```python
from build123d import *

# Parameters (mm, degrees)
SKETCH1_R           = 40
BOSS_EXTRUDE1_DEPTH = 10
SKETCH2_R           = 10
BOSS_EXTRUDE2_DEPTH = 500
SKETCH3_R           = 10
BOSS_EXTRUDE3_DEPTH = 30


with BuildPart() as part:
    # Sketch1 → Boss-Extrude1 (new body)
    with BuildSketch(Plane.XY):
        Circle(SKETCH1_R)
    extrude(amount=BOSS_EXTRUDE1_DEPTH)

    # Sketch2 → Boss-Extrude2 (add)
    with BuildSketch(Plane.XY.offset(10)):
        Circle(SKETCH2_R)
    extrude(amount=BOSS_EXTRUDE2_DEPTH)

    # Sketch3 → Boss-Extrude3 (add)
    with BuildSketch(Plane(origin=(0, 0, 0), x_dir=(-1, 0, 0), z_dir=(0, 0, -1))):
        with Locations((26.998561916, 0)):
            Circle(SKETCH3_R)
    extrude(amount=BOSS_EXTRUDE3_DEPTH)


solid = part.part
```
Model file for the job. Use its own axes, mm. A direction names the side the tool comes from. Coordinates: 2 decimals unless noted, no trailing zeros. Order: outer loops, then holes, each group sorted by start corner. A loop starts at its lowest first (then second) coordinate and runs counter-clockwise, first axis right, second up. Notation, with made-up numbers: M 85,-24.75 L 114,-24.75 A19 ccw 114,-14.75 Z; hole C -22,11 d11. An arc over 180 degrees is marked long. Answer as CSV lines item,"result".
(1) Flat gauge pins, fed straight in: pin 1 (12 mm diameter, centred on y = 2, z = 33, fed in from -X); pin 2 (4 mm diameter, centred on x = 11, y = 6.5, fed in from +Z); pin 3 (3 mm diameter, centred on x = -27, y = -29.5, fed in from -Z). Where does each tip first touch, or does it go through?
Geometry says:
pin 1,"stops at x = -10"
pin 2,"stops at z = 10"
pin 3,"stops at z = 0"
(2) Band-saw the part on B-B, the plane y = 0. List the corners of the cut face in (x, z).
Geometry says:
outline,"M -40,0 L -37,0 L -37,-30 L -17,-30 L -17,0 L 40,0 L 40,10 L 10,10 L 10,510 L -10,510 L -10,10 L -40,10 Z"
(3) Band-saw the part on C-C, the plane z = 249. List the corners of the cut face in (x, y), then the cut area to 3 significant figures.
Geometry says:
outline,"C 0,0 d20"
area,"314 mm2"
(4) Band-saw the part on D-D, the plane x = -29.5. List the corners of the cut face in (y, z), then the cut area to 3 significant figures.
Geometry says:
outline,"M -27.01,0 L -9.68,0 L -9.68,-30 L 9.68,-30 L 9.68,0 L 27.01,0 L 27.01,10 L -27.01,10 Z"
area,"1,120 mm2"
(5) 3-axis set-ups, long thin cutter, end or side, ignore diameter. For faces 1 (the cylindrical face through (-8.67, -39.05, 4.93)), 2 (the flat face through (8, -8, 10)), 3 (the cylindrical face through (-36.54, 3, -14.79)): which of +Z, -Z, +X, -X, +Y, -Y reach the whole face in a straight line?
Geometry says:
face 1,"+Z, -Z"
face 2,"+Z"
face 3,"-Z"
(6) Band-saw the part on A-A, the plane x = 0. List the corners of the cut face in (y, z).
Geometry says:
outline,"M -40,0 L 40,0 L 40,10 L 10,10 L 10,510 L -10,510 L -10,10 L -40,10 Z"
(7) Wall check: line 1 along Z through (x, y) = (-23, -27); line 2 along X through (y, z) = (-6.5, 421); line 3 along Y through (x, z) = (-31.5, 6). Give the ranges that are in metal, low to high.
Geometry says:
line 1,"z = 0 to 10"
line 2,"x = -7.6 to 7.6"
line 3,"y = -24.65 to 24.65"
